Design review of the part built by this model. Coordinates are the model's own, in mm. A direction names the side the tool comes from. Coordinates: 2 decimals unless noted, no trailing zeros. Write each question's results on one line, items separated by ' | '. Start each with the question number.
```python
from build123d import *

# Parameters (mm, degrees)
SKETCH_W     = 11.2
SKETCH_H     = 15.2
PAD_DEPTH    = 10
FILLET_R     = 0.5
FILLET001_R  = 0.2
SKETCH002_R  = 0.590091
POCKET_DEPTH = 1
SKETCH001_W  = 11.2
SKETCH001_H  = 15.2
PAD001_DEPTH = 1.3
CHAMFER_SIZE = 0.1


with BuildPart() as part:
    # Sketch → Pad (new body)
    with BuildSketch(Plane.XY):
        Rectangle(SKETCH_W, SKETCH_H)
    extrude(amount=PAD_DEPTH)

    # Fillet
    fillet_edges = [part.edges().sort_by_distance(p)[0] for p in [
        (-5.6, 0, 10),
        (0, 7.6, 10),
        (5.6, 0, 10),
        (0, -7.6, 10),
        (5.6, -7.6, 5),
        (5.6, 7.6, 5),
        (-5.6, 7.6, 5),
        (-5.6, -7.6, 5),
    ]]
    fillet(fillet_edges, radius=FILLET_R)

    # Fillet001
    fillet001_edges = [part.edges().sort_by_distance(p)[0] for p in [
        (-5.6, 0, 0),
        (-5.453553, -7.453553, 0),
        (-5.453553, 7.453553, 0),
        (0, -7.6, 0),
        (0, 7.6, 0),
        (5.453553, -7.453553, 0),
        (5.453553, 7.453553, 0),
        (5.6, 0, 0),
    ]]
    fillet(fillet001_edges, radius=FILLET001_R)

    # Sketch002 (on Face12 of Fillet001) → Pocket (cut)
    with BuildSketch(Plane.XY.offset(10)):
        with Locations((-3.95892, 5.998271)):
            Circle(SKETCH002_R)
    extrude(amount=-POCKET_DEPTH, mode=Mode.SUBTRACT)

    # Sketch001 (on Face9 of Fillet001) → Pad001 (join)
    with BuildSketch(Plane(origin=(0, 0, 0), x_dir=(1, 0, 0), z_dir=(0, 0, -1))):
        Rectangle(SKETCH001_W, SKETCH001_H)
    extrude(amount=PAD001_DEPTH)

    # Chamfer
    chamfer_edges = [part.edges().sort_by_distance(p)[0] for p in [
        (-4.549011, 5.998271, 10),
    ]]
    chamfer(chamfer_edges, length=CHAMFER_SIZE)


solid = part.part
```
Item 1: For faces 1 (the cylindrical face through (-3.396, 6.176, 9.456)), 2 (the flat face through (-5.6, 0, 5)), list the 3-axis set-ups (+Z, -Z, +X, -X, +Y, -Y) from which the entire face can be reached by the end or side of a thin tool; tool diameter is ignored.
Item 2: Insertion check: pin 1 Ø1.9 at (x, y) = (-3.96, 6) entering from +Z; pin 2 Ø0.9 at (x, y) = (-4, 6) entering from +Z. Each pin has a flat end and moves straight along its axis. Give the tip position at first contact, or say it passes through.
Item 3: Wall thickness on L1, parallel to Y at x = 5.25, z = 7.75: over which ranges is the line inside the solid? List them lowest first.
Item 4: Draft analysis for pull direction Y (two halves, no side actions). For faces 3 (the flat face through (0, -7.6, -1)), 4 (the flat face through (-4, 6, 9)), 5 (the flat face through (5.6, 0, 5)), 6 (the flat face through (0, 7.6, -1)), state which applies: released by +Y, released by -Y, zero draft, split by the parting line, or undercut.
Answer:
1) face 1: +Z | face 2: +Z, -Z, -X, +Y, -Y
2) pin 1: stops at z = 10 | pin 2: stops at z = 9
3) L1: y = -7.58 to 7.58
4) face 3: released by -Y | face 4: undercut | face 5: zero draft | face 6: released by +Y
